```python
from build123d import *

# Parameters (mm, degrees)
F1_DEPTH = 2.54
F2_R     = 6.35
F3_DEPTH = 25.4
F5_DEPTH = 2.54
F6_W     = 18.9905706793
F6_H     = 1.524
F7_DEPTH = 25.4
F8_R     = 1.90499


# Not quite as in the source:
# - a fillet or chamfer is up to 0.001 mm smaller than in the source, because OpenCascade refuses the exact size


with BuildPart() as f1:
    # F0 (on Top) → F1 (new body)
    with BuildSketch(Plane.XY):
        with BuildLine():
            Line((9.8373776994, 27.94), (-9.8373776994, 27.94))
            ThreePointArc((-9.8373776994, 27.94), (-8.5823807234, 19.962322084), (-1.905, 15.4201916351))
            Line((-1.905, 15.4201916351), (-1.905, 25.4))
            Line((-1.905, 25.4), (1.905, 25.4))
            Line((1.905, 25.4), (1.905, 15.4201916351))
            ThreePointArc((1.905, 15.4201916351), (8.5823807234, 19.962322084), (9.8373776994, 27.94))
        make_face()
        with BuildLine():
            Line((-1.905, 25.4), (-1.905, 15.4201916351))
            ThreePointArc((-1.905, 15.4201916351), (0, 15.24), (1.905, 15.4201916351))
            Line((1.905, 15.4201916351), (1.905, 25.4))
            Line((1.905, 25.4), (-1.905, 25.4))
        make_face()
        with BuildLine():
            ThreePointArc((1.905, 15.4201916351), (0, 15.24), (-1.905, 15.4201916351))
            Line((-1.905, 15.4201916351), (-1.905, 5.9228856987))
            ThreePointArc((-1.905, 5.9228856987), (-0.4879681556, 3.1108519733), (0, 0))
            ThreePointArc((0, 0), (0.4879681556, 3.1108519733), (1.905, 5.9228856987))
            Line((1.905, 5.9228856987), (1.905, 15.4201916351))
        make_face()
        with BuildLine():
            ThreePointArc((0, 0), (-0.4879681556, 3.1108519733), (-1.905, 5.9228856987))
            Line((-1.905, 5.9228856987), (-1.905, -5.9228856987))
            ThreePointArc((-1.905, -5.9228856987), (-0.4879681556, -3.1108519733), (0, 0))
        make_face()
        with BuildLine():
            Line((-1.905, -5.9228856987), (-1.905, 5.9228856987))
            ThreePointArc((-1.905, 5.9228856987), (-20.32, 0), (-1.905, -5.9228856987))
        make_face()
        with BuildLine():
            ThreePointArc((20.32, 0), (13.2708519733, 9.6720318444), (1.905, 5.9228856987))
            Line((1.905, 5.9228856987), (1.905, -5.9228856987))
            ThreePointArc((1.905, -5.9228856987), (13.2708519733, -9.6720318444), (20.32, 0))
        make_face()
        with BuildLine():
            Line((1.905, -5.9228856987), (1.905, 5.9228856987))
            ThreePointArc((1.905, 5.9228856987), (0.4879681556, 3.1108519733), (0, 0))
            ThreePointArc((0, 0), (0.4879681556, -3.1108519733), (1.905, -5.9228856987))
        make_face()
        with BuildLine():
            ThreePointArc((0, 0), (-0.4879681556, -3.1108519733), (-1.905, -5.9228856987))
            Line((-1.905, -5.9228856987), (-1.905, -15.4201916351))
            ThreePointArc((-1.905, -15.4201916351), (0, -15.24), (1.905, -15.4201916351))
            Line((1.905, -15.4201916351), (1.905, -5.9228856987))
            ThreePointArc((1.905, -5.9228856987), (0.4879681556, -3.1108519733), (0, 0))
        make_face()
        with BuildLine():
            Line((-1.905, -25.4), (-1.905, -15.4201916351))
            ThreePointArc((-1.905, -15.4201916351), (-8.5823807234, -19.962322084), (-9.8373776994, -27.94))
            Line((-9.8373776994, -27.94), (9.8373776994, -27.94))
            ThreePointArc((9.8373776994, -27.94), (8.5823807234, -19.962322084), (1.905, -15.4201916351))
            Line((1.905, -15.4201916351), (1.905, -25.4))
            Line((1.905, -25.4), (-1.905, -25.4))
        make_face()
        with BuildLine():
            ThreePointArc((1.905, -15.4201916351), (0, -15.24), (-1.905, -15.4201916351))
            Line((-1.905, -15.4201916351), (-1.905, -25.4))
            Line((-1.905, -25.4), (1.905, -25.4))
            Line((1.905, -25.4), (1.905, -15.4201916351))
        make_face()
    extrude(amount=F1_DEPTH)

    # F2 (on face) → F3 (cut)
    with BuildSketch(Plane.XY.offset(2.54)):
        with Locations((0, 25.4)):
            Circle(F2_R)
        with Locations((10.16, 0)):
            Circle(F2_R)
        with Locations((-10.16, 0)):
            Circle(F2_R)
        with Locations((0, -25.4)):
            Circle(F2_R)
    extrude(amount=-F3_DEPTH, mode=Mode.SUBTRACT)

    # F4 (on face) → F5 (join, through all)
    with BuildSketch(Plane.XY.offset(2.54)):
        with BuildLine():
            ThreePointArc((6.35, -17.468852542), (9.1581002397, -21.0005909488), (10.16, -25.4))
            Line((10.16, -25.4), (10.16, -10.16))
            ThreePointArc((10.16, -10.16), (8.2192646134, -9.9729206434), (6.35, -9.4185720786))
            Line((6.35, -9.4185720786), (6.35, -17.468852542))
        make_face()
        with BuildLine():
            ThreePointArc((-10.16, -25.4), (-9.1581002397, -21.0005909488), (-6.35, -17.468852542))
            Line((-6.35, -17.468852542), (-6.35, -9.4185720786))
            ThreePointArc((-6.35, -9.4185720786), (-8.2192646134, -9.9729206434), (-10.16, -10.16))
            Line((-10.16, -10.16), (-10.16, -25.4))
        make_face()
        with BuildLine():
            Line((10.16, 10.16), (10.16, 25.4))
            ThreePointArc((10.16, 25.4), (9.1581002397, 21.0005909488), (6.35, 17.468852542))
            Line((6.35, 17.468852542), (6.35, 9.4185720786))
            ThreePointArc((6.35, 9.4185720786), (8.2192646134, 9.9729206434), (10.16, 10.16))
        make_face()
        with BuildLine():
            ThreePointArc((-6.35, 17.468852542), (-9.1581002397, 21.0005909488), (-10.16, 25.4))
            Line((-10.16, 25.4), (-10.16, 10.16))
            ThreePointArc((-10.16, 10.16), (-8.2192646134, 9.9729206434), (-6.35, 9.4185720786))
            Line((-6.35, 9.4185720786), (-6.35, 17.468852542))
        make_face()
    extrude(amount=-F5_DEPTH)

    # F6 (on face) → F7 (cut)
    with BuildSketch(Plane.XY.offset(2.54)):
        with Locations((19.6552853397, 0)):
            Rectangle(F6_W, F6_H)
        with Locations((-19.6552853397, 0)):
            Rectangle(F6_W, F6_H)
    extrude(amount=-F7_DEPTH, mode=Mode.SUBTRACT)

    # F8 (radius 1.905 in the source; OpenCascade refuses exactly that, so slightly less here)
    f8_edges = [f1.edges().sort_by_distance(p)[0] for p in [
        (20.291385, -0.762, 1.27),
        (20.291385, 0.762, 1.27),
        (16.464114, -0.762, 1.27),
        (16.464114, 0.762, 1.27),
        (5.819871, -27.94, 1.27),
        (-5.819871, -27.94, 1.27),
        (9.837378, -27.94, 1.27),
        (-20.291385, 0.762, 1.27),
        (-20.291385, -0.762, 1.27),
        (-16.464114, -0.762, 1.27),
        (-16.464114, 0.762, 1.27),
        (-9.837378, 27.94, 1.27),
        (5.819871, 27.94, 1.27),
        (-5.819871, 27.94, 1.27),
        (9.837378, 27.94, 1.27),
        (-9.837378, -27.94, 1.27),
    ]]
    fillet(f8_edges, radius=F8_R)


solid = f1.part
```
Check sheet for the modelled part. Datum: model origin and axes. Units: mm. A direction names the side the tool comes from. Round coordinates to 2 decimals unless told otherwise and drop trailing zeros. Loops run counter-clockwise (first coordinate to the right, second up) from the corner with the lowest first, then second, coordinate; pieces in that order, holes last. Notation, with made-up numbers: (80.25, 54) -> (129.25, 54) arc R20 ccw to (129.25, 66) -> close; hole circle Ø11 at (49.5, -13). An arc over 180 degrees is marked (long way). Write item = value, one per line. Start each with the question number.
1) Set-up check for faces 1 (the cylindrical face through (16.878, 1.108, 1.288)), 2 (the cylindrical face through (9.54, -27.42, 1.29)): record each of +Z, -Z, +X, -X, +Y, -Y from which the full face is reachable in a straight line by a thin tool's end or side.
2) Gauge pin test, flat ends, axial feed: pin 1 Ø0.8 at (y, z) = (9.5, 0.5) entering from -X; pin 2 Ø1 at (x, z) = (-14.5, 2) entering from +Y; pin 3 Ø1 at (x, z) = (3.5, 1) entering from +Y. Record the tip position at first contact, or that the pin passes through.
3) Thickness scan on probe 1 along X at (y, z) = (-13, 0.65) (3 decimals); probe 2 along X at (y, z) = (26, 1.25); probe 3 along Y at (x, z) = (-3, 2). Record the ranges inside material, lowest first.
4) Sectioned sample at D-D, the plane z = 1.15. State how many separate pieces and enclosed holes the cut face has, plus the area to 3 significant figures.
5) Sectioned sample at C-C, the plane x = 5. Record the cut outline in (y, z).
6) Release check for a two-part mould opening along X. For faces 3 (the flat face through (-10.16, -18, 1)), 4 (the flat face through (10.16, 18, 1)), 5 (the cylindrical face through (-16.878, -1.108, 1.288)) record: released by +X, released by -X, zero draft, split by the parting line, or undercut.
7) Sectioned sample at A-A, the plane y = 13.5. Record the cut outline in (x, z) (3 decimals), plus the area to 3 significant figures.
8) Sectioned sample at B-B, the plane y = -22.5. Record the cut outline in (x, z), plus the area to 3 significant figures.
Results are:
q1.face_1 = +Z, -Z
q1.face_2 = +Z, -Z, +X, -Y
q2.pin_1 = -14.68
q2.pin_2 = 9.41
q2.pin_3 = 20.47
q3.probe_1 = -10.16 to -6.35, -1.905 to 1.905, 6.35 to 10.16
q3.probe_2 = -10.14 to -6.33, 6.33 to 10.14
q3.probe_3 = -19.8 to -15.69, -7.21 to 7.21, 15.69 to 19.8
q4.separate_pieces = 1
q4.enclosed_holes = 4
q4.area = 844 mm^2
q5.outline = (-21.49, 0) -> (-16.56, 0) -> (-16.56, 2.54) -> (-21.49, 2.54) -> close; (-8.75, 0) -> (-3.7, 0) -> (-3.7, 2.54) -> (-8.75, 2.54) -> close; (3.7, 0) -> (8.75, 0) -> (8.75, 2.54) -> (3.7, 2.54) -> close; (16.56, 0) -> (21.49, 0) -> (21.49, 2.54) -> (16.56, 2.54) -> close
q6.face_3 = released by -X
q6.face_4 = released by +X
q6.face_5 = undercut
q7.outline = (-10.16, 0) -> (-6.35, 0) -> (-6.35, 2.54) -> (-10.16, 2.54) -> close; (-1.905, 0) -> (1.905, 0) -> (1.905, 2.54) -> (-1.905, 2.54) -> close; (6.35, 0) -> (10.16, 0) -> (10.16, 2.54) -> (6.35, 2.54) -> close
q7.area = 29.0 mm^2
q8.outline = (-10.16, 0) -> (-5.65, 0) -> (-5.65, 2.54) -> (-10.16, 2.54) -> close; (5.65, 0) -> (10.16, 0) -> (10.16, 2.54) -> (5.65, 2.54) -> close
q8.area = 22.9 mm^2
